Geometry: final body of the model. Coordinates: model frame, mm. A direction names the side the tool comes from. Round coordinates to 2 decimals unless told otherwise and drop trailing zeros. Loops run counter-clockwise (first coordinate to the right, second up) from the corner with the lowest first, then second, coordinate; pieces in that order, holes last. Notation, with made-up numbers: (75, 22) - (91, 22) arc R21 cw to (91, 49) - close; hole circle Ø4 at (25, 67.5). An arc over 180 degrees is marked (long way). Use CSV: the item, a comma, the result in double quotes.
from build123d import *

# Parameters (mm, degrees)
BOSS_EXTRUDE1_DEPTH = 8
CUT_EXTRUDE2_DEPTH  = 20.5
SKETCH6_W           = 35.270415117
SKETCH6_H           = 22.226622545
CUT_EXTRUDE3_DEPTH  = 8
BOSS_EXTRUDE2_DEPTH = 3
BOSS_EXTRUDE7_DEPTH = 5
SKETCH7_R           = 1.6
CUT_EXTRUDE6_DEPTH  = 40.255572853


with BuildPart() as part:
    # Sketch1 → Boss-Extrude1 (new body)
    with BuildSketch(Plane(origin=(0, 0, 0), x_dir=(0, 0, -1), z_dir=(1, 0, 0))):
        Polygon((0, 0), (0, 16), (-3.5, 16), (-3.5, 4), (-24, 4), (-24, 18), (-31, 18), (-31, 0), align=None)
    boss_extrude1 = extrude(amount=-BOSS_EXTRUDE1_DEPTH)

    # Sketch5 → Cut-Extrude2 (cut)
    with BuildSketch(Plane.XY.offset(3.5)):
        Polygon((-8, 0), (-3, 0), (-5, 4), (-8, 4), align=None)
    cut_extrude2 = extrude(amount=CUT_EXTRUDE2_DEPTH, mode=Mode.SUBTRACT)

    # Mirror1: Boss-Extrude1, Cut-Extrude2 across plane
    add(boss_extrude1.mirror(Plane(origin=(-8, 0, 0), x_dir=(0, 0, 1), z_dir=(1, 0, 0))))
    add(cut_extrude2.mirror(Plane(origin=(-8, 0, 0), x_dir=(0, 0, 1), z_dir=(1, 0, 0))), mode=Mode.SUBTRACT)

    # Sketch6 → Cut-Extrude3 (cut)
    with BuildSketch(Plane(origin=(0, 0, 0), x_dir=(0, 0, -1), z_dir=(1, 0, 0))):
        with Locations((-16.260875851, 8.713036563)):
            Rectangle(SKETCH6_W, SKETCH6_H)
    extrude(amount=-CUT_EXTRUDE3_DEPTH, mode=Mode.SUBTRACT)

    # Sketch9 → Boss-Extrude2 (add)
    with BuildSketch(Plane.XY.offset(3.5)):
        Polygon((-11, 4), (-13, 0), (-8, 0), (-8, 4), align=None)
    extrude(amount=BOSS_EXTRUDE2_DEPTH)

    # Sketch13 → Boss-Extrude7 (add)
    with BuildSketch(Plane.XZ):
        with BuildLine():
            Line((-14, 33), (-6, 33))
            Line((-6, 33), (-6, 26))
            ThreePointArc((-6, 26), (-6.585786438, 24.585786438), (-8, 24))
            Line((-8, 24), (-8, 31))
            Line((-8, 31), (-16, 31))
            ThreePointArc((-16, 31), (-15.414213562, 32.414213562), (-14, 33))
        make_face()
    extrude(amount=-BOSS_EXTRUDE7_DEPTH)

    # Sketch7 → Cut-Extrude6 (cut, through all)
    with BuildSketch(Plane.XY.offset(31)):
        with Locations((-12, 12)):
            Circle(SKETCH7_R)
    extrude(amount=-CUT_EXTRUDE6_DEPTH, mode=Mode.SUBTRACT)


solid = part.part
Item 1: Mould query, pull axis X, two halves, no side actions, for faces 1 (the flat face through (-12, 2, 15)), 2 (the flat face through (-12, 8, 0)), 3 (the cylindrical face through (-15.43, 2.46, 32.4)), 4 (the cylindrical face through (-13.6, 12.07, 1.77)). Classes: released by +X, released by -X, zero draft, split by the parting line, or undercut.
Final values:
face 1,"released by +X"
face 2,"zero draft"
face 3,"released by -X"
face 4,"undercut"
Item 2: Section C-C on y = 5.5. Return the cut outline in (x, z).
Final values:
outline,"(-16, 0) - (-8, 0) - (-8, 3.5) - (-16, 3.5) - close; (-16, 24) - (-8, 24) - (-8, 31) - (-16, 31) - close"
Item 3: Reachability of faces 5 (the flat face through (-12, 10, 3.5)), 6 (the flat face through (-10, 2, 6.5)), 7 (the flat face through (-8, 12, 28)) from +Z, -Z, +X, -X, +Y, -Y: full face, straight path, thin tool, end or side. Return the list, or none.
Final values:
face 5,"+X, -X, +Y"
face 6,"+X, -Y"
face 7,"+Z, -Z, +X, +Y"
Item 4: Material intervals for line 1 (Z direction, x = -8.5, y = 15.75); line 2 (Z direction, x = -9.75, y = 1); line 3 (Y direction, x = -12, z = 27.25), sorted ascending.
Final values:
line 1,"z = 0 to 3.5, 24 to 31"
line 2,"z = 0 to 6.5, 24 to 33"
line 3,"y = 0 to 10.4, 13.6 to 18"
Item 5: Section D-D on y = 11.5. Return the cut outline in (x, z), plus the area to 3 significant figures.
Final values:
outline,"(-16, 0) - (-13.52, 0) - (-13.52, 3.5) - (-16, 3.5) - close; (-16, 24) - (-13.52, 24) - (-13.52, 31) - (-16, 31) - close; (-10.48, 0) - (-8, 0) - (-8, 3.5) - (-10.48, 3.5) - close; (-10.48, 24) - (-8, 24) - (-8, 31) - (-10.48, 31) - close"
area,"52.1 mm²"
Item 6: Section B-B on z = 29.5. Return the cut outline in (x, y), plus the area to 3 significant figures.
Final values:
outline,"(-16, 0) - (-6, 0) - (-6, 5) - (-8, 5) - (-8, 18) - (-16, 18) - close; hole circle Ø3.2 at (-12, 12)"
area,"146 mm²"
Item 7: Pin query (flat end, axial travel): P1, Ø5, axis at x = -12, y = 12, coming from the +Z side; P2, Ø3, axis at x = -12, z = 7.5, coming from the +Y side; P3, Ø5, axis at x = -10, z = 24.5, coming from the -Y side; P4, Ø2, axis at y = 13, z = 27, coming from the +X side. Return the tip coordinate at first contact, or that it passes through.
Final values:
P1,"stops at z = 31"
P2,"stops at y = 4"
P3,"stops at y = 0"
P4,"stops at x = -8"
Item 8: Section A-A on x = -12. Return the cut outline in (y, z), plus the area to 3 significant figures.
Final values:
outline,"(0, 0) - (10.4, 0) - (10.4, 3.5) - (4, 3.5) - (4, 24) - (10.4, 24) - (10.4, 31) - (5, 31) - (5, 33) - (0, 33) - (0, 24) - (2, 24) - (2, 6.5) - (0, 6.5) - close; (13.6, 0) - (16, 0) - (16, 3.5) - (13.6, 3.5) - close; (13.6, 24) - (18, 24) - (18, 31) - (13.6, 31) - close"
area,"205 mm²"
